Design review of the part built by this model. Coordinates are the model's own, in mm. Face numbers are marked on the shaded views. Give positions to 0.01 mm unless a question says otherwise; leave off trailing zeros. Order: outer loops, then holes, each group sorted by start corner. A loop starts at its lowest first (then second) coordinate and runs counter-clockwise, first axis right, second up. Notation, with made-up numbers: (30.5, 83.5) -> (53.5, 83.5) arc R8 ccw to (53.5, 92.5) -> close; hole circle Ø9 at (-9.5, 83). An arc over 180 degrees is marked (long way). Return JSON: item names as keys, results as strings.
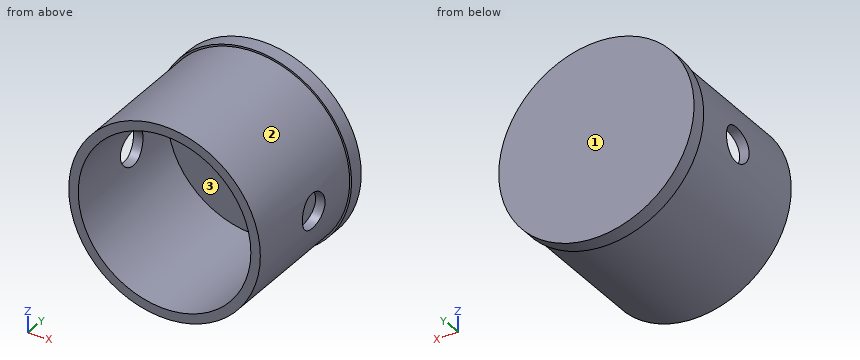
```python
from build123d import *

# Parameters (mm, degrees)
F0_R     = 23.1394
F0_R_2   = 20.850422
F1_DEPTH = 33.243025
F2_R     = 23.588117
F3_DEPTH = 3.598599
F4_R     = 4.212542
F5_DEPTH = 53.346873


with BuildPart() as f1:
    # F0 (on Front) → F1 (new body)
    with BuildSketch(Plane.XZ):
        Circle(F0_R)
        Circle(F0_R_2, mode=Mode.SUBTRACT)
    extrude(amount=F1_DEPTH)

    # F2 (on Front) → F3 (join)
    with BuildSketch(Plane.XZ):
        Circle(F2_R)
    extrude(amount=-F3_DEPTH)

    # F4 (on Right) → F5 (cut, symmetric)
    with BuildSketch(Plane.YZ):
        with Locations((-13.380438, 0)):
            Circle(F4_R)
    extrude(amount=F5_DEPTH, both=True, mode=Mode.SUBTRACT)


solid = f1.part
```
Item 1: Add section B-B (y = -19). Give the boundary of the cut face in (x, z).
Result set:
{"outline": "circle Ø46.28 at (0, 0); hole circle Ø41.7 at (0, 0)"}
Item 2: Add section A-A (z = 0). Give the boundary of the cut face in (x, y), plus the area to 3 significant figures.
Result set:
{"outline": "(-23.59, 0) -> (-23.14, 0) -> (-23.14, -9.17) -> (-20.85, -9.17) -> (-20.85, 0) -> (20.85, 0) -> (20.85, -9.17) -> (23.14, -9.17) -> (23.14, 0) -> (23.59, 0) -> (23.59, 3.6) -> (-23.59, 3.6) -> close; (-23.14, -33.24) -> (-20.85, -33.24) -> (-20.85, -17.59) -> (-23.14, -17.59) -> close; (20.85, -33.24) -> (23.14, -33.24) -> (23.14, -17.59) -> (20.85, -17.59) -> close", "area": "283 mm^2"}
Item 3: Mouldability with a two-part tool opening along X and no side actions: class the marked faces 1, 2 and 3 as released by +X, released by -X, zero draft, split by the parting line, or undercut.
Result set:
{"face 1": "zero draft", "face 2": "split by the parting line", "face 3": "undercut"}
Item 4: Add section D-D (z = -14). Give the boundary of the cut face in (x, y).
Result set:
{"outline": "(-18.98, 0) -> (-18.42, 0) -> (-18.42, -33.24) -> (-15.45, -33.24) -> (-15.45, 0) -> (15.45, 0) -> (15.45, -33.24) -> (18.42, -33.24) -> (18.42, 0) -> (18.98, 0) -> (18.98, 3.6) -> (-18.98, 3.6) -> close"}
Item 5: Wall thickness on L1, parallel to X at y = -20.5, z = 0; L2, parallel to Y at x = 21.75, z = 0; L3, parallel to Z at x = 2, y = -6.5: over which ranges is each line inside the solid? List them lowest first. Write a range as [from, to].
Result set:
{"L1": "x = [-23.14, -20.85], [20.85, 23.14]", "L2": "y = [-33.24, -17.59], [-9.17, 3.6]", "L3": "z = [-23.05, -20.75], [20.75, 23.05]"}
Item 6: Add section C-C (x = 0). Give the boundary of the cut face in (y, z), plus the area to 3 significant figures.
Result set:
{"outline": "(-33.24, -23.14) -> (0, -23.14) -> (0, -23.59) -> (3.6, -23.59) -> (3.6, 23.59) -> (0, 23.59) -> (0, 23.14) -> (-33.24, 23.14) -> (-33.24, 20.85) -> (0, 20.85) -> (0, -20.85) -> (-33.24, -20.85) -> close", "area": "322 mm^2"}
Item 7: For pin 1 (4 mm diameter, centred on x = 4.5, y = -26, fed in from -Z); pin 2 (1.5 mm diameter, centred on x = 8, y = -17.5, fed in from +Z); pin 3 (1.5 mm diameter, centred on y = -11, z = 9, fed in from -X), all flat-tipped, find the tip position at first contact; note any pin that passes through.
Result set:
{"pin 1": "stops at z = -23", "pin 2": "stops at z = 21.97", "pin 3": "stops at x = -21.62"}
